```python
from build123d import *

# Parameters (mm, degrees)
BOSS_EXTRUDE2_DEPTH = 77.5
CHAMFER1_SIZE       = 2
SKETCH2_R           = 2.5
CUT_EXTRUDE1_DEPTH  = 7


with BuildPart() as part:
    # Sketch1 → Boss-Extrude2 (new body)
    with BuildSketch(Plane.XY):
        with BuildLine():
            Line((-8, 8.75), (8, 8.75))
            ThreePointArc((8, 8.75), (9.414213562, 8.164213562), (10, 6.75))
            Line((10, 6.75), (10, 3))
            ThreePointArc((10, 3), (9.707106781, 2.292893219), (9, 2))
            Line((9, 2), (8, 2))
            ThreePointArc((8, 2), (6, 0), (8, -2))
            Line((8, -2), (9, -2))
            Line((9, -2), (22, -2))
            Line((22, -2), (22, 18.75))
            Line((22, 18.75), (-22, 18.75))
            Line((-22, 18.75), (-22, -2))
            Line((-22, -2), (-9, -2))
            Line((-9, -2), (-8, -2))
            ThreePointArc((-8, -2), (-6, 0), (-8, 2))
            Line((-8, 2), (-9, 2))
            ThreePointArc((-9, 2), (-9.707106781, 2.292893219), (-10, 3))
            Line((-10, 3), (-10, 6.75))
            ThreePointArc((-10, 6.75), (-9.414213562, 8.164213562), (-8, 8.75))
        make_face()
    extrude(amount=BOSS_EXTRUDE2_DEPTH)

    # Chamfer1
    chamfer1_edges = [part.edges().sort_by_distance(p)[0] for p in [
        (-22, -2, 38.75),
        (-22, 18.75, 38.75),
        (22, 18.75, 38.75),
        (22, -2, 38.75),
    ]]
    chamfer(chamfer1_edges, length=CHAMFER1_SIZE)

    # Sketch2 → Cut-Extrude1 (cut)
    with BuildSketch(Plane(origin=(0, 18.75, 0), x_dir=(1, 0, 0), z_dir=(0, 1, 0))):
        with Locations(Location((14.728679071, -57.5, 0), (0, 0, 180))):
            Circle(SKETCH2_R)
        with Locations(Location((14.728679071, -20, 0), (0, 0, 180))):
            Circle(SKETCH2_R)
        with Locations((-14.728679071, -57.5)):
            Circle(SKETCH2_R)
        with Locations((-14.728679071, -20)):
            Circle(SKETCH2_R)
    extrude(amount=-CUT_EXTRUDE1_DEPTH, mode=Mode.SUBTRACT)


solid = part.part
```
Work out the finished part from the listing and answer in its coordinate system (mm). A direction names the side the tool comes from. Coordinates: 2 decimals unless noted, no trailing zeros. Loops run counter-clockwise (first coordinate to the right, second up) from the corner with the lowest first, then second, coordinate; pieces in that order, holes last.
1) Section C-C (x = 14.5) is taken. Give the vertices of the cut face in (y, z), plus the area to 3 significant figures.
Results:
outline: (-2, 0) - (18.75, 0) - (18.75, 17.51) - (11.75, 17.51) - (11.75, 22.49) - (18.75, 22.49) - (18.75, 55.01) - (11.75, 55.01) - (11.75, 59.99) - (18.75, 59.99) - (18.75, 77.5) - (-2, 77.5) - close
area: 1,540 mm2
2) Section A-A (y = 7.5) is taken. Give the vertices of the cut face in (x, z).
Results:
outline: (-22, 0) - (-9.85, 0) - (-9.85, 77.5) - (-22, 77.5) - close; (9.85, 0) - (22, 0) - (22, 77.5) - (9.85, 77.5) - close
3) For faces 4 (the flat face through (-21, -1, 38)), 5 (the cylindrical face through (-15.05, 15.3, 17.52)), 6 (the cylindrical face through (-9.43, 8.15, 38.21)), determine the directions among +Z, -Z, +X, -X, +Y, -Y from which every point of the face is accessible in a straight line to the end or side of a thin tool.
Results:
face 4: +Z, -Z, -X, -Y
face 5: +Y
face 6: +Z, -Z
4) A flat-ended cylindrical pin translates along its axis: pin 1 (1.5 mm diameter, centred on x = -13.5, z = 20, fed in from +Y). Find the tip coordinate at first contact, or state that the pin passes through.
Results:
pin 1: stops at y = 11.75
5) For a pull along X with two mould halves and no side action, classify faces 1 (the flat face through (15, 11.75, 20)), 2 (the flat face through (-14, -2, 38)), 3 (the flat face through (22, 8, 38)) as +X half, -X half, draft (parallel to the pull), parting line (faces both ways), or undercut.
Results:
face 1: undercut
face 2: draft
face 3: +X half
6) Section D-D (z = 33.5) is taken. Give the vertices of the cut face in (x, y).
Results:
outline: (-22, 0) - (-20, -2) - (-8, -2) arc R2 ccw to (-8, 2) - (-9, 2) arc R1 cw to (-10, 3) - (-10, 6.75) arc R2 cw to (-8, 8.75) - (8, 8.75) arc R2 cw to (10, 6.75) - (10, 3) arc R1 cw to (9, 2) - (8, 2) arc R2 ccw to (8, -2) - (20, -2) - (22, 0) - (22, 16.75) - (20, 18.75) - (-20, 18.75) - (-22, 16.75) - close
7) Consider probe 1 along X at (y, z) = (0.25, 73); probe 2 along X at (y, z) = (6, 43); probe 3 along Y at (x, z) = (8, 38). Determine where each line is inside the solid, lowest interval first.
Results:
probe 1: x = -22 to -6.02, 6.02 to 22
probe 2: x = -22 to -10, 10 to 22
probe 3: y = -2 to 2, 8.75 to 18.75
8) Section B-B (z = 20) is taken. Give the vertices of the cut face in (x, y), plus the area to 3 significant figures.
Results:
outline: (-22, 0) - (-20, -2) - (-8, -2) arc R2 ccw to (-8, 2) - (-9, 2) arc R1 cw to (-10, 3) - (-10, 6.75) arc R2 cw to (-8, 8.75) - (8, 8.75) arc R2 cw to (10, 6.75) - (10, 3) arc R1 cw to (9, 2) - (8, 2) arc R2 ccw to (8, -2) - (20, -2) - (22, 0) - (22, 16.75) - (20, 18.75) - (17.23, 18.75) - (17.23, 11.75) - (12.23, 11.75) - (12.23, 18.75) - (-12.23, 18.75) - (-12.23, 11.75) - (-17.23, 11.75) - (-17.23, 18.75) - (-20, 18.75) - (-22, 16.75) - close
area: 651 mm2
